Build history of the part. All positions in model axes, mm. Face numbers are marked on the shaded views. A direction names the side the tool comes from. Coordinates: 2 decimals unless noted, no trailing zeros. Write each loop counter-clockwise with the first axis right and the second up, starting at its lowest first coordinate (ties: lowest second). Pieces come first, ordered by that corner, then holes.
from build123d import *

# Parameters (mm, degrees)
SKETCH_1_W          = 450
SKETCH_1_H          = 220
EXTRUDE_1_DEPTH     = 140
SKETCH_2_W          = 450
SKETCH_2_H          = 320
EXTRUDE_2_DEPTH     = 2
SKETCH_3_W          = 444
SKETCH_3_H          = 214
CUT_EXTRUDE_1_DEPTH = 139
SKETCH_4_W          = 444
SKETCH_4_H          = 4
EXTRUDE_3_DEPTH     = 139
SKETCH_5_W          = 60
SKETCH_5_H          = 4
EXTRUDE_4_DEPTH     = 30
SKETCH_6_W          = 137
SKETCH_6_H          = 60
CUT_EXTRUDE_2_DEPTH = 10
SKETCH_7_R          = 7.5
CUT_EXTRUDE_3_DEPTH = 70
SKETCH_8_W          = 2
SKETCH_8_H          = 60
EXTRUDE_5_DEPTH     = 139
SKETCH_9_W          = 30
SKETCH_9_H          = 60
CUT_EXTRUDE_4_DEPTH = 240
SKETCH_10_R         = 7.5
CUT_EXTRUDE_5_DEPTH = 220
SKETCH_11_R         = 7.5
CUT_EXTRUDE_6_DEPTH = 220


with BuildPart() as part:
    # 草图1 → 凸台-拉伸1 (new body)
    with BuildSketch(Plane.XY):
        Rectangle(SKETCH_1_W, SKETCH_1_H)
    extrude(amount=EXTRUDE_1_DEPTH)

    # 草图2 → 凸台-拉伸2 (add)
    with BuildSketch(Plane(origin=(0, 0, 0), x_dir=(-1, 0, 0), z_dir=(0, 0, -1))):
        Rectangle(SKETCH_2_W, SKETCH_2_H)
    extrude(amount=EXTRUDE_2_DEPTH)

    # 草图3 → 切除-拉伸1 (cut)
    with BuildSketch(Plane(origin=(0, 0, -2), x_dir=(-1, 0, 0), z_dir=(0, 0, -1))):
        Rectangle(SKETCH_3_W, SKETCH_3_H)
    extrude(amount=-CUT_EXTRUDE_1_DEPTH, mode=Mode.SUBTRACT)

    # 草图4 → 凸台-拉伸3 (add)
    with BuildSketch(Plane(origin=(0, 0, 137), x_dir=(-1, 0, 0), z_dir=(0, 0, -1))):
        with Locations((0, -32)):
            Rectangle(SKETCH_4_W, SKETCH_4_H)
        with Locations((0, 32)):
            Rectangle(SKETCH_4_W, SKETCH_4_H)
    extrude(amount=EXTRUDE_3_DEPTH)

    # 草图5 → 凸台-拉伸4 (add)
    with BuildSketch(Plane(origin=(0, 0, -2), x_dir=(-1, 0, 0), z_dir=(0, 0, -1))):
        with Locations((-125, 32)):
            Rectangle(SKETCH_5_W, SKETCH_5_H)
        with Locations((-125, -32)):
            Rectangle(SKETCH_5_W, SKETCH_5_H)
    extrude(amount=EXTRUDE_4_DEPTH)

    # 草图6 → 切除-拉伸2 (cut)
    with BuildSketch(Plane(origin=(225, 0, 0), x_dir=(0, 0, -1), z_dir=(1, 0, 0))):
        with Locations((-66.5, 0)):
            Rectangle(SKETCH_6_W, SKETCH_6_H)
    extrude(amount=-CUT_EXTRUDE_2_DEPTH, mode=Mode.SUBTRACT)

    # 草图7 → 切除-拉伸3 (cut)
    with BuildSketch(Plane.XZ.offset(34)):
        with Locations(Location((125, -2, 0), (0, 0, 270))):
            Circle(SKETCH_7_R)
    extrude(amount=-CUT_EXTRUDE_3_DEPTH, mode=Mode.SUBTRACT)

    # 草图8 → 凸台-拉伸5 (add)
    with BuildSketch(Plane(origin=(0, 0, 137), x_dir=(-1, 0, 0), z_dir=(0, 0, -1))):
        with Locations((12, 0)):
            Rectangle(SKETCH_8_W, SKETCH_8_H)
    extrude(amount=EXTRUDE_5_DEPTH)

    # 草图9 → 切除-拉伸4 (cut)
    with BuildSketch(Plane.ZY.offset(225)):
        with Locations((13, 0)):
            Rectangle(SKETCH_9_W, SKETCH_9_H)
    extrude(amount=-CUT_EXTRUDE_4_DEPTH, mode=Mode.SUBTRACT)

    # 草图10 → 切除-拉伸5 (cut)
    with BuildSketch(Plane.XZ.offset(110)):
        with Locations(Location((125, 100, 0), (0, 0, 90))):
            Circle(SKETCH_10_R)
    extrude(amount=-CUT_EXTRUDE_5_DEPTH, mode=Mode.SUBTRACT)

    # 草图11 → 切除-拉伸6 (cut)
    with BuildSketch(Plane.XZ.offset(110)):
        with Locations(Location((-125, 100, 0), (0, 0, 90))):
            Circle(SKETCH_11_R)
    extrude(amount=-CUT_EXTRUDE_6_DEPTH, mode=Mode.SUBTRACT)


solid = part.part
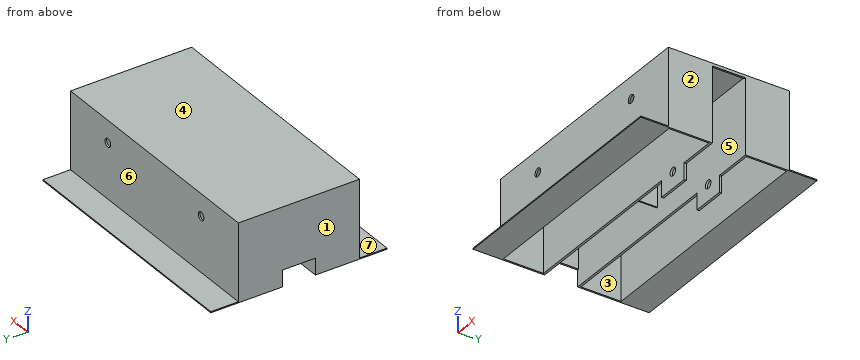
(1) Two-plate mould, pull along X, no slides. Class the marked faces 1, 2, 3 and 4: pulls with the +X half, pulls with the -X half, needs draft (parallel to the pull), parting line crosses it, or undercut.
(2) Flat gauge pins, fed straight in: P1, Ø18, axis at y = -7, z = 92.5, coming from the +X side; P2, Ø1, axis at x = -170.5, z = 38, coming from the +Y side; P3, Ø8, axis at x = 33.5, y = 94, coming from the -Z side. Where does each tip first touch, or does it go through?
(3) Probe L1, parallel to Y at x = 178, z = 75; L2, parallel to X at y = 32.5, z = 100; L3, parallel to X at y = 76.5, z = 86. List the from-to ranges inside material, lowest first.
(4) Slice it at C-C, the plane z = 69.5. List the corners of the cut face in (x, y), and give its area (3 significant figures).
(5) 3-axis set-ups, long thin cutter, end or side, ignore diameter. For the marked faces 5, 6 and 7: which of +Z, -Z, +X, -X, +Y, -Y reach the whole face in a straight line?
(6) Slice it at A-A, the plane y = 101. List the corners of the cut face in (x, z), and give its area (3 significant figures).
(7) Slice it at B-B, the plane x = 28.5. List the corners of the cut face in (y, z).
(8) Slice it at D-D, the plane x = 125. Give the number of separate pieces and of enclosed holes in the cut face, and give its area (3 significant figures).
Results:
1. face 1: pulls with the -X half
1. face 2: pulls with the +X half
1. face 3: undercut
1. face 4: needs draft
2. P1: stops at x = -11
2. P2: stops at y = 110
2. P3: stops at z = 137
3. L1: y = -110 to -107, -34 to -30, 30 to 34, 107 to 110
3. L2: x = -225 to -132.5, -117.5 to 117.5, 132.5 to 225
3. L3: x = -225 to -222, 222 to 225
4. outline: (-225, -110) - (225, -110) - (225, -30) - (-11, -30) - (-11, 30) - (225, 30) - (225, 110) - (-225, 110) - close; hole (-222, -107) - (222, -107) - (222, -34) - (-222, -34) - close; hole (-222, -30) - (-13, -30) - (-13, 30) - (-222, 30) - close; hole (-222, 34) - (222, 34) - (222, 107) - (-222, 107) - close
4. area: 7,480 mm2
5. face 5: -Z
5. face 6: +Z, +X, -X, +Y
5. face 7: +Z, +X, -X, -Y
6. outline: (-225, -2) - (-222, -2) - (-222, 137) - (222, 137) - (222, -2) - (225, -2) - (225, 140) - (-225, 140) - close
6. area: 2,180 mm2
7. outline: (-160, -2) - (-107, -2) - (-107, 137) - (-34, 137) - (-34, -2) - (-30, -2) - (-30, 137) - (30, 137) - (30, -2) - (34, -2) - (34, 137) - (107, 137) - (107, -2) - (160, -2) - (160, 0) - (110, 0) - (110, 140) - (-110, 140) - (-110, 0) - (-160, 0) - close
8. separate pieces: 7
8. enclosed holes: 0
8. area: 2,720 mm2
